```python
from build123d import *

# Parameters (mm, degrees)
SKETCH1_W             = 20
SKETCH1_H             = 10
SKETCH1_R             = 2.6
BOSS_EXTRUDE1_DEPTH   = 3
BOSS_EXTRUDE1_2_DEPTH = 3
SKETCH4_W             = 20
SKETCH4_H             = 62
SKETCH4_R             = 7.5
BOSS_EXTRUDE2_DEPTH   = 3
SKETCH5_W             = 20
SKETCH5_H             = 2.8
BOSS_EXTRUDE3_DEPTH   = 7


with BuildPart() as part:
    # Sketch1 → Boss-Extrude1 (new body)
    with BuildSketch(Plane.XY):
        with Locations((0, 36)):
            Rectangle(SKETCH1_W, SKETCH1_H)
        with Locations((0, 36)):
            Circle(SKETCH1_R, mode=Mode.SUBTRACT)
    extrude(amount=-BOSS_EXTRUDE1_DEPTH)



with BuildPart() as body_2:
    # Sketch1 → Boss-Extrude1 2 (new body)
    with BuildSketch(Plane.XY):
        with Locations((0, -36)):
            Rectangle(SKETCH1_W, SKETCH1_H)
        with Locations((0, -36)):
            Circle(SKETCH1_R, mode=Mode.SUBTRACT)
    extrude(amount=-BOSS_EXTRUDE1_2_DEPTH)


with BuildPart() as body_3:
    # Sketch4 → Boss-Extrude2 (new body)
    with BuildSketch(Plane.XY.offset(-7)):
        Rectangle(SKETCH4_W, SKETCH4_H)
        with Locations((1, 13)):
            Circle(SKETCH4_R, mode=Mode.SUBTRACT)
        with Locations((1, -13)):
            Circle(SKETCH4_R, mode=Mode.SUBTRACT)
    extrude(amount=-BOSS_EXTRUDE2_DEPTH)


with BuildPart() as part_1:
    add(part.part)

    add(body_2.part)  # Boss-Extrude3 merges body 2

    add(body_3.part)  # Boss-Extrude3 merges body 3
    # Sketch5 → Boss-Extrude3 (add)
    with BuildSketch(Plane.XY.offset(-7)):
        with Locations((0, 29.6)):
            Rectangle(SKETCH5_W, SKETCH5_H)
        with Locations((0, -29.6)):
            Rectangle(SKETCH5_W, SKETCH5_H)
    extrude(amount=BOSS_EXTRUDE3_DEPTH)


solid = part_1.part
```
The listing builds one solid part. Answer for the finished solid, in the listing's coordinates (mm). A direction names the side the tool comes from. Give positions to 0.01 mm unless a question says otherwise; leave off trailing zeros. Order: outer loops, then holes, each group sorted by start corner. A loop starts at its lowest first (then second) coordinate and runs counter-clockwise, first axis right, second up. Notation, with made-up numbers: (-39.5, 6.25) - (-25.5, 6.25) arc R11 ccw to (-25.5, 27.25) - close; hole circle Ø1 at (-3, 60). An arc over 180 degrees is marked (long way). Use one line per item in the form item = value. Start each with the question number.
(1) A cutting plane is placed at A-A, the plane z = -2. Write down the section's boundary in (x, y).
(2) A cutting plane is placed at D-D, the plane z = -6.25. Write down the section's boundary in (x, y).
(3) Consider line 1 (Y direction, x = 0, z = -2.3); line 2 (Y direction, x = 1, z = -8.15); line 3 (Y direction, x = 6.75, z = -9). Determine where each line is inside the solid, lowest interval first. Write a range as from..to.
(4) A cutting plane is placed at B-B, the plane x = 1. Write down the section's boundary in (y, z), then the cut area to 3 significant figures.
(5) The mould has two halves that part along X. Classify faces 4 (the cylindrical face through (-0.63, 5.68, -8.48)), 5 (the flat face through (0, 41, -1)), 6 (the flat face through (-10, 0, -8)): released by +X, released by -X, zero draft, split by the parting line, or undercut.
(6) A cutting plane is placed at C-C, the plane y = -13. Write down the section's boundary in (x, z), then the cut area to 3 significant figures.
(7) Flat-ended cylindrical pins translate along their axes: pin 1 Ø6 at (x, y) = (1, 1) entering from +Z; pin 2 Ø2 at (x, y) = (-2, -19.5) entering from -Z; pin 3 Ø5 at (x, y) = (-2.5, 36.5) entering from -Z; pin 4 Ø3.5 at (x, z) = (-1.5, -7.5) entering from -Y. Find the tip coordinate at first contact, or state that the pin passes through.
(8) For faces 1 (the flat face through (0, 31, -7)), 2 (the flat face through (-2, -34, -3)), 3 (the flat face through (0, -28.2, -4)), determine the directions among +Z, -Z, +X, -X, +Y, -Y from which every point of the face is accessible in a straight line to the end or side of a thin tool.
Ans:
q1.outline = (-10, -41) - (10, -41) - (10, -28.2) - (-10, -28.2) - close; (-10, 28.2) - (10, 28.2) - (10, 41) - (-10, 41) - close; hole circle Ø5.2 at (0, -36); hole circle Ø5.2 at (0, 36)
q2.outline = (-10, -31) - (10, -31) - (10, -28.2) - (-10, -28.2) - close; (-10, 28.2) - (10, 28.2) - (10, 31) - (-10, 31) - close
q3.line_1 = -41..-38.6, -33.4..-28.2, 28.2..33.4, 38.6..41
q3.line_2 = -31..-20.5, -5.5..5.5, 20.5..31
q3.line_3 = -31..-17.82, -8.18..8.18, 17.82..31
q4.outline = (-41, -3) - (-38.4, -3) - (-38.4, 0) - (-41, 0) - close; (-33.6, -3) - (-31, -3) - (-31, -10) - (-20.5, -10) - (-20.5, -7) - (-28.2, -7) - (-28.2, 0) - (-33.6, 0) - close; (-5.5, -10) - (5.5, -10) - (5.5, -7) - (-5.5, -7) - close; (20.5, -10) - (31, -10) - (31, -3) - (33.6, -3) - (33.6, 0) - (28.2, 0) - (28.2, -7) - (20.5, -7) - close; (38.4, -3) - (41, -3) - (41, 0) - (38.4, 0) - close
q4.area = 166 mm^2
q5.face_4 = undercut
q5.face_5 = zero draft
q5.face_6 = released by -X
q6.outline = (-10, -10) - (-6.5, -10) - (-6.5, -7) - (-10, -7) - close; (8.5, -10) - (10, -10) - (10, -7) - (8.5, -7) - close
q6.area = 15.0 mm^2
q7.pin_1 = -7
q7.pin_2 = -10
q7.pin_3 = -3
q7.pin_4 = -31
q8.face_1 = -Z, +X, -X, +Y
q8.face_2 = -Z, +X, -X, -Y
q8.face_3 = +Z, +X, -X
